```python
from build123d import *

# Parameters (mm, degrees)
F0_R     = 7.9375
F0_R_2   = 5.715
F1_DEPTH = 12.7


with BuildPart() as f1:
    # F0 (on Top) → F1 (new body)
    with BuildSketch(Plane.XY):
        with BuildLine():
            ThreePointArc((-17.690877, -6.35), (-18.796, 0), (-17.690877, 6.35))
            Line((-17.690877, 6.35), (-22.225, 6.35))
            ThreePointArc((-22.225, 6.35), (-24.470064, 5.420064), (-25.4, 3.175))
            Line((-25.4, 3.175), (-25.4, -3.175))
            ThreePointArc((-25.4, -3.175), (-24.470064, -5.420064), (-22.225, -6.35))
            Line((-22.225, -6.35), (-17.690877, -6.35))
        make_face()
        with BuildLine():
            ThreePointArc((17.690877, -6.35), (18.517658, -3.222724), (18.796, 0))
            ThreePointArc((18.796, 0), (18.517658, 3.222724), (17.690877, 6.35))
            ThreePointArc((17.690877, 6.35), (13.290779, 13.290779), (6.35, 17.690877))
            ThreePointArc((6.35, 17.690877), (0, 18.796), (-6.35, 17.690877))
            ThreePointArc((-6.35, 17.690877), (-13.290779, 13.290779), (-17.690877, 6.35))
            ThreePointArc((-17.690877, 6.35), (-18.796, 0), (-17.690877, -6.35))
            ThreePointArc((-17.690877, -6.35), (-13.290779, -13.290779), (-6.35, -17.690877))
            ThreePointArc((-6.35, -17.690877), (0, -18.796), (6.35, -17.690877))
            ThreePointArc((6.35, -17.690877), (13.290779, -13.290779), (17.690877, -6.35))
        make_face()
        Circle(F0_R, mode=Mode.SUBTRACT)
        with BuildLine():
            ThreePointArc((-6.35, 17.690877), (0, 18.796), (6.35, 17.690877))
            Line((6.35, 17.690877), (6.35, 22.225))
            ThreePointArc((6.35, 22.225), (5.420064, 24.470064), (3.175, 25.4))
            Line((3.175, 25.4), (-3.175, 25.4))
            ThreePointArc((-3.175, 25.4), (-5.420064, 24.470064), (-6.35, 22.225))
            Line((-6.35, 22.225), (-6.35, 17.690877))
        make_face()
        with BuildLine():
            Line((6.35, -22.225), (6.35, -17.690877))
            ThreePointArc((6.35, -17.690877), (0, -18.796), (-6.35, -17.690877))
            Line((-6.35, -17.690877), (-6.35, -22.225))
            ThreePointArc((-6.35, -22.225), (-5.420064, -24.470064), (-3.175, -25.4))
            Line((-3.175, -25.4), (3.175, -25.4))
            ThreePointArc((3.175, -25.4), (5.420064, -24.470064), (6.35, -22.225))
        make_face()
        with BuildLine():
            ThreePointArc((17.690877, 6.35), (18.517658, 3.222724), (18.796, 0))
            ThreePointArc((18.796, 0), (18.517658, -3.222724), (17.690877, -6.35))
            Line((17.690877, -6.35), (22.225, -6.35))
            ThreePointArc((22.225, -6.35), (24.470064, -5.420064), (25.4, -3.175))
            Line((25.4, -3.175), (25.4, 3.175))
            ThreePointArc((25.4, 3.175), (24.470064, 5.420064), (22.225, 6.35))
            Line((22.225, 6.35), (17.690877, 6.35))
        make_face()
        Circle(F0_R)
        Circle(F0_R_2, mode=Mode.SUBTRACT)
    extrude(amount=F1_DEPTH)


solid = f1.part
```
The model under review builds one solid part; all positions refer to its coordinate system, in mm. A direction names the side the tool comes from. Give positions to 0.01 mm unless a question says otherwise; leave off trailing zeros. Write each loop counter-clockwise with the first axis right and the second up, starting at its lowest first coordinate (ties: lowest second). Pieces come first, ordered by that corner, then holes. Notation, with made-up numbers: (-3, 46) - (29, 46) arc R25 ccw to (29, 68) - close; hole circle Ø11 at (20, 40.25). An arc over 180 degrees is marked (long way). Answer in a Markdown table with one row per item. Add a question column.
1. Tool access review of faces 4 (the flat face through (6.35, 20, 6)), 5 (the flat face through (20, -6.35, 6)), 6 (the flat face through (-6, 0, 12.7)), 7 (the cylindrical face through (-24.45, 5.44, 6.26)), 8 (the flat face through (-6.35, -20, 6)): name each direction out of +Z, -Z, +X, -X, +Y, -Y from which nothing blocks a thin tool from reaching the whole face with its end or side.
2. We need section C-C on z = 5.5. Write out the cut boundary in (x, y) (3 decimals), then the cut area to 3 significant figures.
3. Draft analysis for pull direction Y (two halves, no side actions). For faces 1 (the flat face through (6.35, -20, 6)), 2 (the cylindrical face through (5.44, 24.45, 6.26)), 3 (the cylindrical face through (5.45, 1.72, 6.26)), state which applies: +Y half, -Y half, draft (parallel to the pull), parting line (faces both ways), or undercut.
4. Wall thickness on line 1 along Y through (x, z) = (0, 3) (3 decimals); line 2 along X through (y, z) = (-22, 8.5): over which ranges is each line inside the solid? List them lowest first. Write a range as [from, to].
5. Insertion check: P1, Ø3.5, axis at x = 19, z = 4, coming from the -Y side; P2, Ø1.4, axis at y = -19, z = 9, coming from the +X side; P3, Ø3, axis at x = 9, z = 3.5, coming from the -Y side. Each pin has a flat end and moves straight along its axis. Give the tip position at first contact, or say it passes through.
6. We need section D-D on x = 21. Write out the cut boundary in (y, z), then the cut area to 3 significant figures.
7. We need section A-A on y = 0. Write out the cut boundary in (x, z) (3 decimals), then the cut area to 3 significant figures.
Ans:
| question | item | result |
|---|---|---|
| 1 | face 4 | +Z, -Z, +X, +Y |
| 1 | face 5 | +Z, -Z, +X, -Y |
| 1 | face 6 | +Z, +X, -X, +Y, -Y |
| 1 | face 7 | +Z, -Z, -X, +Y |
| 1 | face 8 | +Z, -Z, -X, -Y |
| 2 | outline | (-25.4, -3.175) arc R3.175 ccw to (-22.225, -6.35) - (-17.691, -6.35) arc R18.796 ccw to (-6.35, -17.691) - (-6.35, -22.225) arc R3.175 ccw to (-3.175, -25.4) - (3.175, -25.4) arc R3.175 ccw to (6.35, -22.225) - (6.35, -17.691) arc R18.796 ccw to (17.691, -6.35) - (22.225, -6.35) arc R3.175 ccw to (25.4, -3.175) - (25.4, 3.175) arc R3.175 ccw to (22.225, 6.35) - (17.691, 6.35) arc R18.796 ccw to (6.35, 17.691) - (6.35, 22.225) arc R3.175 ccw to (3.175, 25.4) - (-3.175, 25.4) arc R3.175 ccw to (-6.35, 22.225) - (-6.35, 17.691) arc R18.796 ccw to (-17.691, 6.35) - (-22.225, 6.35) arc R3.175 ccw to (-25.4, 3.175) - close; hole circle Ø11.43 at (0, 0) |
| 2 | area | 1,340 mm^2 |
| 3 | face 1 | draft |
| 3 | face 2 | +Y half |
| 3 | face 3 | undercut |
| 4 | line 1 | y = [-25.4, -5.715], [5.715, 25.4] |
| 4 | line 2 | x = [-6.35, 6.35] |
| 5 | P1 | stops at y = -7.47 |
| 5 | P2 | stops at x = 6.35 |
| 5 | P3 | stops at y = -17.23 |
| 6 | outline | (-6.35, 0) - (6.35, 0) - (6.35, 12.7) - (-6.35, 12.7) - close |
| 6 | area | 161 mm^2 |
| 7 | outline | (-25.4, 0) - (-5.715, 0) - (-5.715, 12.7) - (-25.4, 12.7) - close; (5.715, 0) - (25.4, 0) - (25.4, 12.7) - (5.715, 12.7) - close |
| 7 | area | 500 mm^2 |
